from build123d import *

# Parameters (mm, degrees)
F2_R     = 17.272
F3_DEPTH = 5.08
F4_SIZE  = 1.524
F5_R     = 2.413
F6_R     = 12.7


with BuildPart() as f1:
    # F0 (on Front) → F1 (revolve)
    with BuildSketch(Plane.XZ):
        Polygon((0, 5.08), (0, 0), (47.2628956169, 0), (52.3428956169, 0), (52.3428956169, 67.6072314382), (33.2928956169, 67.6072314382), (33.2928956169, 76.8034979701), (28.2128956169, 76.8034979701), (28.2128956169, 62.5348), (47.2628956169, 62.5348), (47.2628956169, 5.08), align=None)
    revolve(axis=Axis((0, 0, 38.4017489851), (0, 0, 1)))

    # F2
    f2_edges = [f1.edges().sort_by_distance(p)[0] for p in [
        (-52.342896, 0, 67.607231),
    ]]
    fillet(f2_edges, radius=F2_R)

    # F3 (add): a face of the model
    f3_faces = [f1.faces().sort_by_distance(p)[0] for p in [
        (-32.3512303266, 0, 76.8034979701),
    ]]
    extrude(f3_faces, amount=F3_DEPTH)

    # F4
    f4_edges = [f1.edges().sort_by_distance(p)[0] for p in [
        (-28.212896, 0, 81.883498),
        (-33.292896, 0, 81.883498),
    ]]
    chamfer(f4_edges, length=F4_SIZE)

    # F5
    f5_edges = [f1.edges().sort_by_distance(p)[0] for p in [
        (-31.768896, 0, 81.883498),
        (-29.736896, 0, 81.883498),
    ]]
    fillet(f5_edges, radius=F5_R)

    # F6
    f6_edges = [f1.edges().sort_by_distance(p)[0] for p in [
        (-28.212896, 0, 62.5348),
    ]]
    fillet(f6_edges, radius=F6_R)


solid = f1.part
Model file for the job. Use its own axes, mm. A direction names the side the tool comes from. Give positions to 0.01 mm unless a question says otherwise; leave off trailing zeros. Loops run counter-clockwise (first coordinate to the right, second up) from the corner with the lowest first, then second, coordinate; pieces in that order, holes last.
1) Flat gauge pins, fed straight in: pin 1 Ø8 at (x, z) = (29, 30.5) entering from -Y; pin 2 Ø6 at (y, z) = (-32.5, 34) entering from -X; pin 3 Ø8 at (x, y) = (33, -4.5) entering from -Z; pin 4 Ø5 at (x, z) = (0.5, 33.5) entering from +Y. Where does each tip first touch, or does it go through?
2) Tool access for faces 1 (the cylindrical face through (-11.347, -51.098, 25.52)), 2 (the flat face through (31, -13, 67.607)), 3 (the flat face through (14, 39, 62.535)): list every direction of +Z, -Z, +X, -X, +Y, -Y with a clear straight run to the whole face (end or side of a thin tool).
3) Saw through at C-C (z = 12). Write the cut outline in (x, y), plus the area to 3 significant figures.
4) Pull direction X, two halves, no side cores. Call faces 4 (the conical face through (15, -29, 81)), 5 (the cylindrical face through (-3.673, 27.973, 77.761)), 6 (the flat face through (1, 1, 0)): +X half, -X half, draft (parallel to the pull), parting line (faces both ways), or undercut.
5) Wall check: line 1 (Y direction, x = 0, z = 39); line 2 (Y direction, x = -20.5, z = 72); line 3 (Z direction, x = 26.5, y = 19.5). Give the ranges that are in metal, low to high.
6) Saw through at D-D (z = 54). Write the cut outline in (x, y), plus the area to 3 significant figures.
Answer block:
1. pin 1: stops at y = -45.99
1. pin 2: stops at x = -43.24
1. pin 3: stops at z = 0
1. pin 4: stops at y = 52.34
2. face 1: +Z, -Z
2. face 2: +Z
2. face 3: none
3. outline: circle Ø104.69 at (0, 0); hole circle Ø94.53 at (0, 0)
3. area: 1,590 mm2
4. face 4: parting line
4. face 5: undercut
4. face 6: draft
5. line 1: y = -52.34 to -47.26, 47.26 to 52.34
5. line 2: y = -26.23 to -19.99, 19.99 to 26.23
5. line 3: z = 0 to 5.08, 65.38 to 80.75
6. outline: circle Ø103.9 at (0, 0); hole circle Ø94.53 at (0, 0)
6. area: 1,460 mm2
